from build123d import *

# Parameters (mm, degrees)
SKETCH1_R           = 25
BOSS_EXTRUDE1_DEPTH = 12
CHAMFER1_SIZE       = 0.5
BOSS_EXTRUDE2_DEPTH = 13
SKETCH4_R           = 4.25
CUT_EXTRUDE1_DEPTH  = 6
CIRPATTERN1_COUNT   = 5


# Read off the part's stored shape, not the designer's step: Boss-Extrude2
with BuildPart() as part:
    # Sketch1 → Boss-Extrude1 (new body)
    with BuildSketch(Plane.XY):
        Circle(SKETCH1_R)
    extrude(amount=BOSS_EXTRUDE1_DEPTH)

    # Chamfer1
    chamfer1_edges = [part.edges().sort_by_distance(p)[0] for p in [
        (-25, 0, 12),
    ]]
    chamfer(chamfer1_edges, length=CHAMFER1_SIZE)

    # Boss-Extrude2 outline → Boss-Extrude2 (add)
    with BuildSketch(Plane.XY.offset(12)):
        with BuildLine():
            ThreePointArc((-21.046908053, 12.541039089), (-12.609472348, 8.942183166), (-7, 16.2))
            Line((-7, 16.2), (-7, 20))
            Line((-7, 20), (-14.150971698, 20))
            ThreePointArc((-14.150971698, 20), (-17.989766791, 16.631845682), (-21.046908053, 12.541039089))
        make_face()
    extrude(amount=BOSS_EXTRUDE2_DEPTH)

    # Sketch4 → Cut-Extrude1 (cut)
    with BuildSketch(Plane(origin=(0, 0, 0), x_dir=(-1, 0, 0), z_dir=(0, 0, -1))):
        with Locations((0, 17.5)):
            Circle(SKETCH4_R)
    cut_extrude1 = extrude(amount=-CUT_EXTRUDE1_DEPTH, mode=Mode.SUBTRACT)

    # CirPattern1: Cut-Extrude1 ×5 about axis
    cirpattern1_axis = Axis((0, 0, 0), (0, 0, 1))
    for i in range(1, CIRPATTERN1_COUNT):
        add(cut_extrude1.rotate(cirpattern1_axis, i * 360 / CIRPATTERN1_COUNT), mode=Mode.SUBTRACT)


solid = part.part
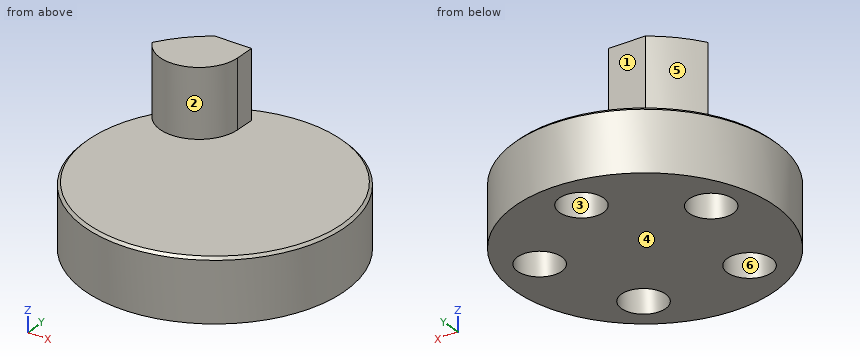
Input: part model. Units: mm. Frame: model coordinates. Face numbers are marked on the shaded views. A direction names the side the tool comes from. Round coordinates to 2 decimals unless told otherwise and drop trailing zeros. Order: outer loops, then holes, each group sorted by start corner. A loop starts at its lowest first (then second) coordinate and runs counter-clockwise, first axis right, second up. Notation, with made-up numbers: (-31.5, 60.25) - (-22.5, 60.25) arc R13 cw to (-22.5, 71.25) - close; hole circle Ø8 at (64.25, 80). An arc over 180 degrees is marked (long way). Use a Markdown table: item, result.
1. Access query for the marked faces 1, 2 and 3. Directions: +Z, -Z, +X, -X, +Y, -Y. A direction counts if a zero-diameter tool reaches every point of the face in a straight line with its end or side. Return the directions, or none.
Evaluation:
| item | result |
|---|---|
| face 1 | +Z, +X, -X, +Y |
| face 2 | +Z, -Y |
| face 3 | -Z |
2. Section B-B on y = 0. Return the cut outline in (x, z), then the cut area to 3 significant figures.
Evaluation:
| item | result |
|---|---|
| outline | (-25, 0) - (25, 0) - (25, 11.5) - (24.5, 12) - (-24.5, 12) - (-25, 11.5) - close |
| area | 600 mm^2 |
3. Mould query, pull axis X, two halves, no side actions, for the marked faces 4, 5 and 6. Classes: +X half, -X half, draft (parallel to the pull), parting line (faces both ways), or undercut.
Evaluation:
| item | result |
|---|---|
| face 4 | draft |
| face 5 | -X half |
| face 6 | undercut |
4. Section A-A on x = 0. Return the cut outline in (y, z), then the cut area to 3 significant figures.
Evaluation:
| item | result |
|---|---|
| outline | (-25, 0) - (13.25, 0) - (13.25, 6) - (21.75, 6) - (21.75, 0) - (25, 0) - (25, 11.5) - (24.5, 12) - (-24.5, 12) - (-25, 11.5) - close |
| area | 549 mm^2 |
5. First-contact query: pin 1 (7.5 mm diameter, centred on x = -10.29, y = -14.16, fed in from +Z); pin 2 (5 mm diameter, centred on x = -16.5, z = 19.5, fed in from +Y); pin 3 (6 mm diameter, centred on y = -3, z = 14, fed in from -X). Flat tips, straight axial feed; report the tip coordinate or a pass-through.
Evaluation:
| item | result |
|---|---|
| pin 1 | z = 12 |
| pin 2 | y = 20 |
| pin 3 | x = -24.96 |
6. Section D-D on z = 19.25. Return the cut outline in (x, y).
Evaluation:
| item | result |
|---|---|
| outline | (-21.05, 12.54) arc R7.5 ccw to (-7, 16.2) - (-7, 20) - (-14.15, 20) arc R24.5 ccw to start |
7. Material intervals for probe 1 along Y at (x, z) = (0, 4.7); probe 2 along Y at (x, z) = (14, 3.75); probe 3 along Y at (x, z) = (-13, 3.25), sorted ascending.
Evaluation:
| item | result |
|---|---|
| probe 1 | -25 to 13.25, 21.75 to 25 |
| probe 2 | -20.71 to -16.22, -12.09 to 2.08, 8.74 to 20.71 |
| probe 3 | -21.35 to -17.43, -10.89 to 3.22, 7.6 to 21.35 |
8. Section C-C on z = 8.5. Return the cut outline in (x, y).
Evaluation:
| item | result |
|---|---|
| outline | circle Ø50 at (0, 0) |
